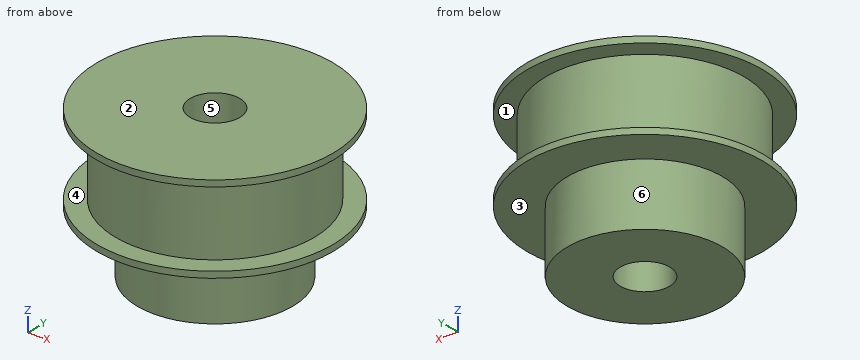
Autodesk Inventor part; units mm, degrees
ref_plane "YZ Plane" through (0, 0, 0) normal (1, 0, 0) x (0, 1, 0)
ref_plane "XZ Plane" through (0, 0, 0) normal (0, 1, 0) x (-1, 0, 0)
ref_plane "XY Plane" through (0, 0, 0) normal (0, 0, 1) x (1, 0, 0)
sketch "Sketch1" plane through (0, 0, 0) normal (0, 0, 1) x (1, 0, 0)
  circle A0 centre (0, 0) radius 12.5
  dimension "d0" = 25
extrude "Extrusion1" add sketch "Sketch1" along normal blind 10
sketch "Sketch2" plane through (0, 0, 10) normal (0, 0, 1) x (1, 0, 0)
  circle A0 centre (0, 0) radius 19
  dimension "d3" = 38
extrude "Extrusion2" add sketch "Sketch2" along normal blind 1
sketch "Sketch3" plane through (0, 0, 11) normal (0, 0, 1) x (1, 0, 0)
  circle A0 centre (0, 0) radius 16
  dimension "d6" = 32
extrude "Extrusion3" add sketch "Sketch3" along normal blind 12
sketch "Sketch4" plane through (0, 0, 23) normal (0, 0, 1) x (1, 0, 0)
  circle A0 centre (0, 0) radius 19
  dimension "d9" = 38
extrude "Extrusion4" add sketch "Sketch4" along normal blind 1
sketch "Sketch5" plane through (0, 0, 24) normal (0, 0, 1) x (1, 0, 0)
  circle A0 centre (0, 0) radius 4
  dimension "d12" = 8
extrude "Extrusion5" cut sketch "Sketch5" against normal through all
properties part number "Pulley"
Can you work these out from the model? Positions are in its coordinate system, mm. Face numbers are marked on the shaded views. A direction names the side the tool comes from. Coordinates: 2 decimals unless noted, no trailing zeros. Order: outer loops, then holes, each group sorted by start corner. A loop starts at its lowest first (then second) coordinate and runs counter-clockwise, first axis right, second up. Notation, with made-up numbers: M 7.5,2 L 14.5,2 A26 ccw 14.5,40 Z; hole C -39.75,37 d10. An arc over 180 degrees is marked long. Write item = value, one per line.
(1) For pin 1 Ø2 at (x, y) = (-11.5, -14) entering from -Z; pin 2 Ø3 at (x, z) = (0.5, 7) entering from +Y; pin 3 Ø10 at (x, z) = (10, 3) entering from +Y, each with a flat end and sliding along its axis, tell me the tip position at first contact or that it passes through.
Results are:
pin_1 = 10
pin_2 = 12.5
pin_3 = 11.46
(2) Suppose I cut it at D-D on y = 6.5. Please give me the cut outline in (x, z), plus the area to 3 significant figures.
Results are:
outline = M -17.85,10 L -10.68,10 L -10.68,0 L 10.68,0 L 10.68,10 L 17.85,10 L 17.85,11 L 14.62,11 L 14.62,23 L 17.85,23 L 17.85,24 L -17.85,24 L -17.85,23 L -14.62,23 L -14.62,11 L -17.85,11 Z
area = 636 mm2
(3) If we mould it in two halves opening along X, with no side actions, what happens to the marked faces 4, 5 and 6? For each: pulls with the +X half, pulls with the -X half, needs draft (parallel to the pull), parting line crosses it, or undercut.
Results are:
face_4 = needs draft
face_5 = undercut
face_6 = parting line crosses it
(4) I need wall thicknesses on line 1 along Y through (x, z) = (0, 8); line 2 along Y through (x, z) = (0, 13.75); line 3 along Z through (x, y) = (-8, 13.5). Which ranges of each line are inside material? Lowest first, please. Write a range as [from, to].
Results are:
line_1 = [-12.5, -4], [4, 12.5]
line_2 = [-16, -4], [4, 16]
line_3 = [10, 24]
(5) Suppose I cut it at C-C on z = 17.5. Please give me the cut outline in (x, y), plus the area to 3 significant figures.
Results are:
outline = C 0,0 d32; hole C 0,0 d8
area = 754 mm2
(6) Suppose I cut it at A-A on y = 0. Please give me the cut outline in (x, z), plus the area to 3 significant figures.
Results are:
outline = M -19,10 L -12.5,10 L -12.5,0 L -4,0 L -4,24 L -19,24 L -19,23 L -16,23 L -16,11 L -19,11 Z; M 4,0 L 12.5,0 L 12.5,10 L 19,10 L 19,11 L 16,11 L 16,23 L 19,23 L 19,24 L 4,24 Z
area = 518 mm2
(7) For the marked faces 1, 2 and 3, which set-ups out of +Z, -Z, +X, -X, +Y, -Y let a thin tool reach every point of the face, with its end or its side?
Results are:
face_1 = none
face_2 = +Z, +X, -X, +Y, -Y
face_3 = -Z
